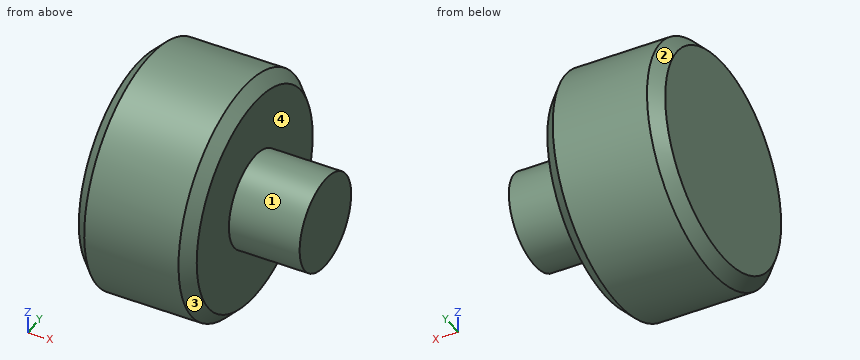
Autodesk Inventor part; units mm, degrees
ref_plane "YZ Plane" through (0, 0, 0) normal (1, 0, 0) x (0, 1, 0)
ref_plane "XZ Plane" through (0, 0, 0) normal (0, 1, 0) x (-1, 0, 0)
ref_plane "XY Plane" through (0, 0, 0) normal (0, 0, 1) x (1, 0, 0)
sketch "スケッチ1" plane through (0, 0, 0) normal (0, 1, 0) x (-1, 0, 0)
  line L0 (-5.0796, -45.5704) -> (-5.0796, 73.9296)
  line L1 (-5.0796, 73.9296) -> (-4.5796, 74.4296)
  line L2 (-4.5796, 74.4296) -> (24.4204, 74.4296)
  line L3 (24.4204, 74.4296) -> (24.9204, 73.9296)
  line L4 (24.9204, 73.9296) -> (24.9204, -45.5704)
  line L5 (24.9204, -45.5704) -> (-5.0796, -45.5704)
  line L6 (1.9204, -47.0704) -> (1.9204, -50.5704)
  line L7 (1.9204, -50.5704) -> (17.9204, -50.5704)
  line L8 (17.9204, -50.5704) -> (17.9204, -47.0704)
  line L9 (17.9204, -47.0704) -> (1.9204, -47.0704)
  line L10 (2.9204, -47.0704) -> (2.9204, -45.5704)
  line L11 (16.9204, -45.5704) -> (16.9204, -47.0704)
  line L12 (31.4204, 56.4296) -> (30.9204, 56.9296)
  line L13 (30.9204, 56.9296) -> (30.9204, 71.9296)
  line L14 (30.9204, 71.9296) -> (31.4204, 72.4296)
  line L15 (31.4204, 72.4296) -> (38.4204, 72.4296)
  line L16 (38.4204, 72.4296) -> (38.9204, 71.9296)
  line L17 (38.9204, 71.9296) -> (38.9204, 56.9296)
  line L18 (38.9204, 56.9296) -> (38.4204, 56.4296)
  line L19 (38.4204, 56.4296) -> (31.4204, 56.4296)
  line L20 (31.4204, 56.4296) -> (31.4204, 72.4296)
  line L21 (30.9204, 70.4296) -> (27.9204, 70.4296)
  line L22 (27.9204, 70.4296) -> (27.9204, 58.4296)
  line L23 (27.9204, 58.4296) -> (30.9204, 58.4296)
  line L24 (38.4204, 56.4296) -> (38.4204, 72.4296)
  line L25 (27.9204, 66.9296) -> (24.9204, 66.9296)
  line L26 (27.4204, 66.9296) -> (27.4204, 61.9296)
  line L27 (27.9204, 61.9296) -> (24.9204, 61.9296)
  line L28 (24.9204, 73.9296) -> (-5.0796, 73.9296)
  line L29 (-5.0796, 97.1797) -> (24.9204, 97.1797)
  line L30 (24.9204, 97.1797) -> (24.9204, 105.1797)
  line L31 (24.9204, 105.1797) -> (-5.0796, 105.1797)
  line L32 (-5.0796, 105.1797) -> (-5.0796, 97.1797)
  line L33 (24.9204, 99.1797) -> (27.9204, 99.1797)
  line L34 (27.2723, 99.1797) -> (27.2723, 103.1797)
  line L35 (27.9204, 103.1797) -> (24.9204, 103.1797)
  line L36 (27.9204, 105.6797) -> (27.9204, 96.6797)
  line L37 (27.9204, 96.6797) -> (28.4204, 96.1797)
  line L38 (28.4204, 96.1797) -> (32.4204, 96.1797)
  line L39 (32.4204, 96.1797) -> (32.9204, 96.6797)
  line L40 (32.9204, 96.6797) -> (32.9204, 105.6797)
  line L41 (32.9204, 105.6797) -> (32.4204, 106.1797)
  line L42 (32.4204, 106.1797) -> (28.4204, 106.1797)
  line L43 (28.4204, 106.1797) -> (27.9204, 105.6797)
  line L44 (28.4204, 106.1797) -> (28.4204, 96.1797)
  line L45 (32.4204, 96.1797) -> (32.4204, 106.1797)
  line L46 (2.4204, -50.5704) -> (2.4204, -47.0704)
  line L47 (-0.0796, -40.5704) -> (-0.0796, 74.4296)
  line L48 (19.9204, 74.4296) -> (19.9204, -40.5704)
  line L49 (19.9204, -40.5704) -> (9.9204, -46.3439)
  line L50 (9.9204, -46.3439) -> (-0.0796, -40.5704)
  line L51 (-0.0796, -40.5704) -> (19.9204, -40.5704)
  line L52 (17.4204, -47.0704) -> (17.4204, -50.5704)
  line L53 (9.9204, -56.5156) -> (9.9204, 78.76)
  line L54 (9.9204, 93.5864) -> (9.9204, 108.5157)
  line L55 (19.9204, 105.1797) -> (19.9204, 97.1797)
  line L56 (22.5096, 101.1797) -> (35.2156, 101.1797)
  line L57 (27.9204, 103.1797) -> (27.2723, 102.4797)
  line L58 (27.2723, 102.4797) -> (24.9204, 102.4797)
  line L59 (24.9204, 99.8797) -> (27.2723, 99.8797)
  line L60 (27.2723, 99.8797) -> (27.9204, 99.1797)
  line L61 (-0.0796, 97.1797) -> (-0.0796, 105.1797)
  line L62 (24.9204, 66.2296) -> (27.4204, 66.2296)
  line L63 (27.4204, 66.2296) -> (27.9204, 66.9296)
  line L64 (27.4204, 62.6296) -> (27.9204, 61.9296)
  line L65 (27.4204, 62.6296) -> (24.9204, 62.6296)
  line L66 (22.6428, 64.4296) -> (42.5049, 64.4296)
  line L67 (32.2954, 71.4296) -> (38.4204, 71.4296)
  line L68 (33.1704, 70.4296) -> (38.4204, 70.4296)
  line L69 (34.0454, 69.4296) -> (38.4204, 69.4296)
  line L70 (34.9204, 68.4296) -> (38.4204, 68.4296)
  line L71 (35.7954, 67.4296) -> (38.4204, 67.4296)
  line L72 (36.6704, 66.4296) -> (38.4204, 66.4296)
  line L73 (37.5454, 65.4296) -> (38.4204, 65.4296)
  line L74 (29.2204, 105.1797) -> (32.4204, 105.1797)
  line L75 (30.0204, 104.1797) -> (32.4204, 104.1797)
  line L76 (30.8204, 103.1797) -> (32.4204, 103.1797)
  line L77 (31.6204, 102.1797) -> (32.4204, 102.1797)
  point P0 (0, 0)
  point P1 (52.3578, -69.094)
  point P2 (52.3578, -59.2279)
  point P3 (24.9204, 101.1797)
  point P4 (32.9204, 101.1797)
revolve "回転1" add sketch "スケッチ1" angle 360 about axis through (-22.5096, 0, 101.1797) along (-1, 0, 0) contours L35 L34 L58 L30 | L30 L58 L34 L56 | L35 L57 L34 | L34 L57 L36 L56 | L36 L43 L44 L56 | L44 L42 L45 L56 | L45 L41 L40 L56
thread "ねじ1"
properties part number "ring_handle" material "アルミニウム 6061"
Source: CAD feature listing. Evaluate the final solid. Frame: model axes, mm. Face numbers are marked on the shaded views. A direction names the side the tool comes from. Round coordinates to 2 decimals unless told otherwise and drop trailing zeros. Loops run counter-clockwise (first coordinate to the right, second up) from the corner with the lowest first, then second, coordinate; pieces in that order, holes last. Notation, with made-up numbers: (-40, -39) - (2, -39) arc R34 cw to (2, -4) - close; hole circle Ø1 at (47.5, 82.5). An arc over 180 degrees is marked (long way). Write item = value, one per line. Start each with the question number.
Item 1: First-contact query: pin 1 Ø1.5 at (x, y) = (-27, -2.5) entering from +Z; pin 2 Ø1.5 at (x, y) = (-27.5, 3.5) entering from -Z; pin 3 Ø1.5 at (x, z) = (-30.5, 103) entering from +Y. Flat tips, straight axial feed; report the tip coordinate or a pass-through.
Item 2: Material intervals for line 1 (X direction, y = 0, z = 104); line 2 (X direction, y = 2, z = 97); line 3 (Y direction, x = -28.5, z = 97), sorted ascending.
Item 3: Reachability of the marked faces 1 and 2 from +Z, -Z, +X, -X, +Y, -Y: full face, straight path, thin tool, end or side. Return the list, or none.
Item 4: Mould query, pull axis Z, two halves, no side actions, for the marked faces 3 and 4. Classes: released by +Z, released by -Z, zero draft, split by the parting line, or undercut.
Item 5: Section query A-A on y = 0. Output: boundary loops of the cut face in (x, z).
Item 6: Section query B-B on x = -28.75. Output: boundary loops of the cut face in (y, z), plus the area to 3 significant figures.
Item 7: Section query C-C on x = -26.75. Output: boundary loops of the cut face in (y, z).
Results list:
q1.pin_1 = 102.15
q1.pin_2 = 97.63
q1.pin_3 = 4.88
q2.line_1 = -32.92 to -27.92
q2.line_2 = -32.79 to -28.05
q2.line_3 = -2.74 to 2.74
q3.face_1 = +X
q3.face_2 = -X
q4.face_3 = split by the parting line
q4.face_4 = zero draft
q5.outline = (-32.92, 96.68) - (-32.42, 96.18) - (-28.42, 96.18) - (-27.92, 96.68) - (-27.92, 99.18) - (-24.92, 99.18) - (-24.92, 103.18) - (-27.92, 103.18) - (-27.92, 105.68) - (-28.42, 106.18) - (-32.42, 106.18) - (-32.92, 105.68) - close
q6.outline = circle Ø10 at (0, 101.18)
q6.area = 78.5 mm²
q7.outline = circle Ø4 at (0, 101.18)
